Check sheet for the modelled part. Datum: model origin and axes. Units: mm. A direction names the side the tool comes from. Coordinates: 2 decimals unless noted, no trailing zeros. Loops run counter-clockwise (first coordinate to the right, second up) from the corner with the lowest first, then second, coordinate; pieces in that order, holes last. Notation, with made-up numbers: (-33.75, -38.75) - (5.25, -38.75) arc R10 cw to (5.25, -22.75) - close; hole circle Ø7 at (-17.75, -37). An arc over 180 degrees is marked (long way). Answer as a JSON object with one key per item and string values. Group by question number.
from build123d import *


with BuildPart() as part:
    # Sketch1 → Revolve1 (revolve)
    with BuildSketch(Plane.XY, mode=Mode.PRIVATE) as revolve1_sk:
        with BuildLine():
            Line((0, 40), (0, 37))
            Line((0, 37), (8, 37))
            ThreePointArc((8, 37), (9.414213562, 36.414213562), (10, 35))
            Line((10, 35), (10, 2))
            Line((10, 2), (13, 2))
            Line((13, 2), (13, 35))
            ThreePointArc((13, 35), (13.585786438, 36.414213562), (15, 37))
            Line((15, 37), (18, 37))
            Line((18, 37), (18, 50))
            ThreePointArc((18, 50), (18.585786438, 51.414213562), (20, 52))
            Line((20, 52), (48, 52))
            Line((48, 52), (48, 55))
            Line((48, 55), (18, 55))
            Line((18, 55), (18, 60))
            Line((18, 60), (15, 60))
            Line((15, 60), (15, 52))
            Line((15, 52), (15, 40))
            Line((15, 40), (0, 40))
        make_face()
    revolve(revolve1_sk.sketch.rotate(Axis((0, 0, 0), (1, 0, 0)), 90), axis=Axis((0, 0, 0), (1, 0, 0)))


solid = part.part
1. Material ranges on line 1 (Y direction, x = 35.5, z = 0); line 2 (Y direction, x = 15.9, z = 0); line 3 (X direction, y = -18, z = 10.5), recorded low to high.
2. Release check for a two-part mould opening along Z. For faces 1 (the face through (18, -37.3, 0.2)), 2 (the face through (13, 7, 0)), 3 (the face through (32.79, 48.794, 25.379)), 4 (the face through (18, 49, -26)) record: released by +Z, released by -Z, zero draft, split by the parting line, or undercut.
3. Sectioned sample at C-C on x = 6.5. Record the cut outline in (y, z), plus the area to 3 significant figures.
4. Gauge pin test, flat ends, axial feed: pin 1 (12 mm diameter, centred on x = 19.5, z = 33.5, fed in from -Y); pin 2 (1.5 mm diameter, centred on x = 8, z = -26.5, fed in from +Y); pin 3 (6 mm diameter, centred on x = 33, y = -22.5, fed in from -Z). Record the tip position at first contact, or that the pin passes through.
5. Sectioned sample at D-D on x = 43.5. Record the cut outline in (y, z).
6. Access from +Z, -Z, +X, -X, +Y, -Y to the whole of each face (thin tool, end or side, straight path). Record for faces 5 (the face through (16.521, 32.825, 17.073)), 6 (the face through (48, 20, -49)), 7 (the face through (4.056, 32.825, 17.073)).
Answers follow:
{
 "1": {"line 1": "y = -55 to -52, 52 to 55", "line 2": "y = -60 to -37, 37 to 60", "line 3": "x = 10 to 13"},
 "2": {"face 1": "undercut", "face 2": "undercut", "face 3": "split by the parting line", "face 4": "zero draft"},
 "3": {"outline": "circle Ø80 at (0, 0); hole circle Ø74 at (0, 0)", "area": "726 mm^2"},
 "4": {"pin 1": "stops at y = -53.23", "pin 2": "stops at y = 30.61", "pin 3": "stops at z = -51.43"},
 "5": {"outline": "circle Ø110 at (0, 0); hole circle Ø104 at (0, 0)"},
 "6": {"face 5": "+X", "face 6": "+Z, -Z, +X, +Y, -Y", "face 7": "-X"}
}
